Build history of the part. All positions in model axes, mm. A direction names the side the tool comes from. Give positions to 0.01 mm unless a question says otherwise; leave off trailing zeros. Loops run counter-clockwise (first coordinate to the right, second up) from the corner with the lowest first, then second, coordinate; pieces in that order, holes last. Notation, with made-up numbers: M 71,84 L 106,84 A15 cw 106,107 Z; hole C 0.5,85 d7. An arc over 180 degrees is marked long. Answer as a JSON object with one key per item and string values. Group by question number.
1. Slice it at A-A (z = 0). List the corners of the cut face in (x, y), then the cut area to 4 significant figures.
2. Drill centre lines: line 1 along Z through (x, y) = (9, 9); line 2 along Z through (x, y) = (-10.05, 47.8); line 3 along X through (y, z) = (2, 36.5). Where is each one in solid material? Low to high. Write a range as [from, to].
3. Slice it at B-B (y = 35). List the corners of the cut face in (x, z), then the cut area to 4 significant figures.
4. 3-axis set-ups, long thin cutter, end or side, ignore diameter. For faces 5 (the face through (60.5, 23, -1)), 6 (the face through (-18.938, 48.835, 40.025)): which of +Z, -Z, +X, -X, +Y, -Y reach the whole face in a straight line?
5. Slice it at C-C (x = 28). List the corners of the cut face in (y, z), then the cut area to 3 significant figures.
6. Mould opens along Z. For faces 1 (the face through (-1, 25, -53)), 2 (the face through (29, 51.3, -23)), 3 (the face through (-60.5, 23, 1)), 4 (the face through (1, 25, 53)) say: released by +Z, released by -Z, zero draft, split by the parting line, or undercut.
7. Drop a flat-ended pin along its axis: pin 1 Ø1.2 at (x, z) = (-4.5, 51.5) entering from -Y. Give the stop position or say it passes through.
8. Slice it at D-D (x = -54). List the corners of the cut face in (y, z).
Autodesk Inventor part; units mm, degrees
ref_plane "YZ Plane" through (0, 0, 0) normal (1, 0, 0) x (0, 1, 0)
ref_plane "XZ Plane" through (0, 0, 0) normal (0, 1, 0) x (-1, 0, 0)
ref_plane "XY Plane" through (0, 0, 0) normal (0, 0, 1) x (1, 0, 0)
sketch "Sketch1" plane through (0, 0, 0) normal (0, 1, 0) x (-1, 0, 0)
  line L0 (63, -53) -> (-63, -53)
  line L1 (-63, -53) -> (-63, 53)
  line L2 (-63, 53) -> (63, 53)
  line L3 (63, 53) -> (63, -53)
  point P0 (0, 0)
  point P1 (63, 0)
  point P2 (0, -53)
  dimension "d0" = 126
  dimension "d1" = 106
extrude "Extrusion1" add sketch "Sketch1" along normal blind 51.3
sketch "Sketch2" plane through (0, 0, 0) normal (0, -1, 0) x (1, 0, 0)
  line L0 (60.5, 50.5) -> (-60.5, 50.5)
  line L1 (-60.5, 50.5) -> (-60.5, -50.5)
  line L2 (-60.5, -50.5) -> (60.5, -50.5)
  line L3 (60.5, -50.5) -> (60.5, 50.5)
  line L4 (63, 53) -> (63, -53)
  line L5 (-63, 53) -> (63, 53)
  point P0 (0, 0)
  point P1 (60.5, 0)
  point P2 (0, 50.5)
  dimension "d8" = 2.5
  dimension "d9" = 2.5
extrude "Extrusion2" cut sketch "Sketch2" against normal blind 46.3
sketch "Sketch3" plane through (0, 51.3, 0) normal (0, 1, 0) x (1, 0, 0)
  circle A0 centre (-10.05, 0) radius 41
  line L0 (63, -53) -> (63, 53)
  point P0 (0, 0)
  point P1 (63, 0)
  dimension "d12" = 82
  dimension "d13" = 73.05
extrude "Extrusion3" cut sketch "Sketch3" against normal blind 46.3
sketch "Sketch4" plane through (-63, 0, 53) normal (0, 0, 1) x (1, 0, 0)
  line L0 (37.95, 24.425) -> (42.95, 24.425)
  line L1 (42.95, 24.425) -> (42.95, 15.625)
  line L2 (42.95, 15.625) -> (37.95, 15.625)
  line L3 (37.95, 15.625) -> (37.95, 24.425)
  line L4 (0, 0) -> (126, 0)
  line L5 (0, 0) -> (0, 51.3)
  line L6 (52.95, 22.525) -> (61.75, 22.525)
  line L7 (61.75, 22.525) -> (61.75, 17.525)
  line L8 (61.75, 17.525) -> (52.95, 17.525)
  line L9 (52.95, 17.525) -> (52.95, 22.525)
  point P0 (63, 0)
  point P1 (57.35, 17.525)
  point P2 (40.45, 15.625)
  point P3 (42.95, 20.025)
  point P4 (52.95, 20.025)
  dimension "d16" = 5
  dimension "d17" = 8.8
  dimension "d18" = 15.625
  dimension "d19" = 37.95
  dimension "d20" = 8.8
  dimension "d21" = 5
  dimension "d22" = 10
extrude "Extrusion4" cut sketch "Sketch4" against normal blind 10
equation "\"d20\" = d17"
equation "\"d21\" = d16"
properties part number "Bottom_Cover"
Established:
{
 "1": {"outline": "M -63,0 L -60.5,0 L -60.5,46.3 L -51.05,46.3 L -51.05,51.3 L -63,51.3 Z; M 30.95,46.3 L 60.5,46.3 L 60.5,0 L 63,0 L 63,51.3 L 30.95,51.3 Z", "area": "451.5 mm^2"},
 "2": {"line 1": "z = [-53, -50.5], [50.5, 53]", "line 2": "z = [-53, -41], [41, 53]", "line 3": "x = [-63, -60.5], [60.5, 63]"},
 "3": {"outline": "M -63,-53 L 63,-53 L 63,53 L -63,53 Z; hole M -60.5,-50.5 L 60.5,-50.5 L 60.5,50.5 L -60.5,50.5 Z", "area": "1,135 mm^2"},
 "4": {"face 5": "-Y", "face 6": "+Y, -Y"},
 "5": {"outline": "M 0,-53 L 51.3,-53 L 51.3,-15.27 L 46.3,-15.27 L 46.3,-50.5 L 0,-50.5 Z; M 0,50.5 L 46.3,50.5 L 46.3,15.27 L 51.3,15.27 L 51.3,53 L 0,53 Z", "area": "609 mm^2"},
 "6": {"face 1": "released by -Z", "face 2": "zero draft", "face 3": "undercut", "face 4": "released by +Z"},
 "7": {"pin 1": "stops at y = 0"},
 "8": {"outline": "M 0,-53 L 51.3,-53 L 51.3,53 L 0,53 L 0,50.5 L 46.3,50.5 L 46.3,-50.5 L 0,-50.5 Z"}
}
